Geometry check sheet. Reference: the model listing, model coordinates, mm. Face numbers are marked on the shaded views. A direction names the side the tool comes from. Round coordinates to 2 decimals unless told otherwise and drop trailing zeros. Order: outer loops, then holes, each group sorted by start corner. A loop starts at its lowest first (then second) coordinate and runs counter-clockwise, first axis right, second up. Notation, with made-up numbers: (-23, -9) - (-8, -9) arc R11 cw to (-8, -4) - close; hole circle Ø9 at (17, -17.5). An arc over 180 degrees is marked (long way). Use a Markdown table: item, result. Add a question column.
(1) Section check B-B on z = -10.5. Record the boundary of the cut face in (x, y), then the cut area to 3 significant figures.
(2) Section check C-C on x = -9.5. Record the boundary of the cut face in (y, z), then the cut area to 3 significant figures.
(3) Section check A-A on y = -8.75. Record the boundary of the cut face in (x, z).
(4) Section check D-D on z = -2. Record the boundary of the cut face in (x, y), then the cut area to 3 significant figures.
(5) Access from +Z, -Z, +X, -X, +Y, -Y to the whole of each face (thin tool, end or side, straight path). Record for the marked faces 1, 2, 3, 4 and 5.
(6) Mould release check, pull along X, two halves, no side actions. Record for the marked faces 6, 7 and 8: released by +X, released by -X, zero draft, split by the parting line, or undercut.
(7) Gauge pin test, flat ends, axial feed: P1, Ø11.5, axis at x = 5.5, z = 1, coming from the -Y side; P2, Ø6, axis at x = -13.5, y = -11, coming from the +Z side; P3, Ø5, axis at x = 8, y = -9, coming from the -Z side; P4, Ø5.5, axis at y = -9, z = 10.5, coming from the -X side. Record the tip position at first contact, or that the pin passes through.
(8) Thickness scan on line 1 along X through (y, z) = (-7.5, 11); line 2 along X through (y, z) = (-4, 2). Record the ranges inside material, lowest first. Write a range as [from, to].
```python
from build123d import *

# Parameters (mm, degrees)
F1_DEPTH     = 2.032
F2_DEPTH     = 12.7
F3_T1_DEPTH  = 21.463
F3_T3_DEPTH  = 21.463
F3_T5_DEPTH  = 20.574
F3_T7_DEPTH  = 21.463
F3_T9_DEPTH  = 20.574
F3_T11_DEPTH = 21.463
F3_T17_DEPTH = 27.813
F3_T21_DEPTH = 27.813
F3_T28_DEPTH = 27.813
F3_T32_DEPTH = 27.813
F3_T39_DEPTH = 27.813
F3_T43_DEPTH = 27.813
F3_T50_DEPTH = 27.813
F3_T54_DEPTH = 27.813


# Not quite as in the source:
# - a fillet or chamfer that OpenCascade refuses, or shapes differently, is made with other operations: its cross-section is extruded or revolved along the edge and cut away or added


with BuildPart() as f1:
    # F0 (on Front) → F1 (new body)
    with BuildSketch(Plane.XZ):
        Polygon((1.397, 19.05), (-1.397, 19.05), (-1.397, 1.397), (-19.05, 1.397), (-19.05, -1.397), (-1.397, -1.397), (-1.397, -19.05), (1.397, -19.05), (1.397, -1.397), (19.05, -1.397), (19.05, 1.397), (1.397, 1.397), align=None)
    extrude(amount=F1_DEPTH)

    # F0 (on Front) → F2 (join)
    with BuildSketch(Plane.XZ):
        Polygon((-1.397, 19.05), (-3.937, 19.05), (-3.937, 3.937), (-19.05, 3.937), (-19.05, 1.397), (-1.397, 1.397), align=None)
        Polygon((3.937, 19.05), (1.397, 19.05), (1.397, 1.397), (19.05, 1.397), (19.05, 3.937), (3.937, 3.937), align=None)
        Polygon((-1.397, -1.397), (-19.05, -1.397), (-19.05, -3.937), (-3.937, -3.937), (-3.937, -19.05), (-1.397, -19.05), align=None)
        Polygon((19.05, -3.937), (19.05, -1.397), (1.397, -1.397), (1.397, -19.05), (3.937, -19.05), (3.937, -3.937), align=None)
    extrude(amount=F2_DEPTH)

    # F3: fillet of radius 2.54 on 12 edges, made by hand

    # F3_s2 → F3_t1 (cut)
    with BuildSketch(Plane.XY.offset(3.937)):
        with BuildLine():
            ThreePointArc((-3.937, -2.54), (-3.1930512242, -0.7439487758), (-1.397, 0))
            Line((-1.397, 0), (-3.937, 0))
            Line((-3.937, 0), (-3.937, -2.54))
        make_face()
        with BuildLine():
            ThreePointArc((3.937, -2.54), (3.1930512242, -0.7439487758), (1.397, 0))
            Line((1.397, 0), (3.937, 0))
            Line((3.937, 0), (3.937, -2.54))
        make_face()
    extrude(amount=F3_T1_DEPTH, mode=Mode.SUBTRACT)

    # F3_s4 → F3_t3 (cut)
    with BuildSketch(Plane.YZ.offset(-25.4)):
        with BuildLine():
            ThreePointArc((-2.54, 3.937), (-0.7439487758, 3.1930512242), (0, 1.397))
            Line((0, 1.397), (0, 3.937))
            Line((0, 3.937), (-2.54, 3.937))
        make_face()
        with BuildLine():
            ThreePointArc((-2.54, -3.937), (-0.7439487758, -3.1930512242), (0, -1.397))
            Line((0, -1.397), (0, -3.937))
            Line((0, -3.937), (-2.54, -3.937))
        make_face()
    extrude(amount=F3_T3_DEPTH, mode=Mode.SUBTRACT)

    # F3_s6 → F3_t5 (cut)
    with BuildSketch(Plane.XY.offset(-10.287)):
        with BuildLine():
            ThreePointArc((-19.05, -2.54), (-18.3060512242, -0.7439487758), (-16.51, 0))
            Line((-16.51, 0), (-19.05, 0))
            Line((-19.05, 0), (-19.05, -2.54))
        make_face()
        with BuildLine():
            ThreePointArc((19.05, -2.54), (18.3060512242, -0.7439487758), (16.51, 0))
            Line((16.51, 0), (19.05, 0))
            Line((19.05, 0), (19.05, -2.54))
        make_face()
    extrude(amount=F3_T5_DEPTH, mode=Mode.SUBTRACT)

    # F3_s8 → F3_t7 (cut)
    with BuildSketch(Plane.XY.offset(-25.4)):
        with BuildLine():
            ThreePointArc((-3.937, -2.54), (-3.1930512242, -0.7439487758), (-1.397, 0))
            Line((-1.397, 0), (-3.937, 0))
            Line((-3.937, 0), (-3.937, -2.54))
        make_face()
        with BuildLine():
            ThreePointArc((3.937, -2.54), (3.1930512242, -0.7439487758), (1.397, 0))
            Line((1.397, 0), (3.937, 0))
            Line((3.937, 0), (3.937, -2.54))
        make_face()
    extrude(amount=F3_T7_DEPTH, mode=Mode.SUBTRACT)

    # F3_s10 → F3_t9 (cut)
    with BuildSketch(Plane.YZ.offset(-10.287)):
        with BuildLine():
            ThreePointArc((-2.54, -19.05), (-0.7439487758, -18.3060512242), (0, -16.51))
            Line((0, -16.51), (0, -19.05))
            Line((0, -19.05), (-2.54, -19.05))
        make_face()
        with BuildLine():
            ThreePointArc((-2.54, 19.05), (-0.7439487758, 18.3060512242), (0, 16.51))
            Line((0, 16.51), (0, 19.05))
            Line((0, 19.05), (-2.54, 19.05))
        make_face()
    extrude(amount=F3_T9_DEPTH, mode=Mode.SUBTRACT)

    # F3_s12 → F3_t11 (cut)
    with BuildSketch(Plane.YZ.offset(3.937)):
        with BuildLine():
            ThreePointArc((-2.54, -3.937), (-0.7439487758, -3.1930512242), (0, -1.397))
            Line((0, -1.397), (0, -3.937))
            Line((0, -3.937), (-2.54, -3.937))
        make_face()
        with BuildLine():
            ThreePointArc((-2.54, 3.937), (-0.7439487758, 3.1930512242), (0, 1.397))
            Line((0, 1.397), (0, 3.937))
            Line((0, 3.937), (-2.54, 3.937))
        make_face()
    extrude(amount=F3_T11_DEPTH, mode=Mode.SUBTRACT)


with BuildPart() as f3_tool15:
    # F3_s16 → F3_t17 (new body)
    with BuildSketch(Plane.XY.offset(25.4)):
        with BuildLine():
            ThreePointArc((-3.937, -2.54), (-3.1930512242, -0.7439487758), (-1.397, 0))
            Line((-1.397, 0), (-3.937, 0))
            Line((-3.937, 0), (-3.937, -2.54))
        make_face()
    extrude(amount=-F3_T17_DEPTH)

    split(bisect_by=Plane.XY.offset(3.937), keep=Keep.BOTTOM)


with BuildPart() as f3_tool19:
    # F3_s20 → F3_t21 (new body)
    with BuildSketch(Plane.YZ.offset(2.413)):
        with BuildLine():
            ThreePointArc((-2.54, 3.937), (-0.7439487758, 3.1930512242), (0, 1.397))
            Line((0, 1.397), (0, 3.937))
            Line((0, 3.937), (-2.54, 3.937))
        make_face()
    extrude(amount=-F3_T21_DEPTH)

    split(bisect_by=Plane.YZ.offset(-3.937), keep=Keep.TOP)


with BuildPart() as f3_tool15_1:
    add(f3_tool15.part)

    # F3_t23: intersect F3_tool19
    add(f3_tool19.part, mode=Mode.INTERSECT)


with BuildPart() as f1_1:
    add(f1.part)

    # F3_t13: cut F3_tool15
    add(f3_tool15_1.part, mode=Mode.SUBTRACT)


with BuildPart() as f3_tool26:
    # F3_s27 → F3_t28 (new body)
    with BuildSketch(Plane.YZ.offset(-25.4)):
        with BuildLine():
            ThreePointArc((-2.54, -3.937), (-0.7439487758, -3.1930512242), (0, -1.397))
            Line((0, -1.397), (0, -3.937))
            Line((0, -3.937), (-2.54, -3.937))
        make_face()
    extrude(amount=F3_T28_DEPTH)

    split(bisect_by=Plane.YZ.offset(-3.937), keep=Keep.TOP)


with BuildPart() as f3_tool30:
    # F3_s31 → F3_t32 (new body)
    with BuildSketch(Plane.XY.offset(2.413)):
        with BuildLine():
            ThreePointArc((-3.937, -2.54), (-3.1930512242, -0.7439487758), (-1.397, 0))
            Line((-1.397, 0), (-3.937, 0))
            Line((-3.937, 0), (-3.937, -2.54))
        make_face()
    extrude(amount=-F3_T32_DEPTH)

    split(bisect_by=Plane.XY.offset(-3.937), keep=Keep.TOP)


with BuildPart() as f3_tool26_1:
    add(f3_tool26.part)

    # F3_t34: intersect F3_tool30
    add(f3_tool30.part, mode=Mode.INTERSECT)


with BuildPart() as f1_2:
    add(f1_1.part)

    # F3_t24: cut F3_tool26
    add(f3_tool26_1.part, mode=Mode.SUBTRACT)


with BuildPart() as f3_tool37:
    # F3_s38 → F3_t39 (new body)
    with BuildSketch(Plane.XY.offset(-25.4)):
        with BuildLine():
            ThreePointArc((3.937, -2.54), (3.1930512242, -0.7439487758), (1.397, 0))
            Line((1.397, 0), (3.937, 0))
            Line((3.937, 0), (3.937, -2.54))
        make_face()
    extrude(amount=F3_T39_DEPTH)

    split(bisect_by=Plane.XY.offset(-3.937), keep=Keep.TOP)


with BuildPart() as f3_tool41:
    # F3_s42 → F3_t43 (new body)
    with BuildSketch(Plane.YZ.offset(-2.413)):
        with BuildLine():
            ThreePointArc((-2.54, -3.937), (-0.7439487758, -3.1930512242), (0, -1.397))
            Line((0, -1.397), (0, -3.937))
            Line((0, -3.937), (-2.54, -3.937))
        make_face()
    extrude(amount=F3_T43_DEPTH)

    split(bisect_by=Plane.YZ.offset(3.937), keep=Keep.BOTTOM)


with BuildPart() as f3_tool37_1:
    add(f3_tool37.part)

    # F3_t45: intersect F3_tool41
    add(f3_tool41.part, mode=Mode.INTERSECT)


with BuildPart() as f1_3:
    add(f1_2.part)

    # F3_t35: cut F3_tool37
    add(f3_tool37_1.part, mode=Mode.SUBTRACT)


with BuildPart() as f3_tool48:
    # F3_s49 → F3_t50 (new body)
    with BuildSketch(Plane.YZ.offset(25.4)):
        with BuildLine():
            ThreePointArc((-2.54, 3.937), (-0.7439487758, 3.1930512242), (0, 1.397))
            Line((0, 1.397), (0, 3.937))
            Line((0, 3.937), (-2.54, 3.937))
        make_face()
    extrude(amount=-F3_T50_DEPTH)

    split(bisect_by=Plane.YZ.offset(3.937), keep=Keep.BOTTOM)


with BuildPart() as f3_tool52:
    # F3_s53 → F3_t54 (new body)
    with BuildSketch(Plane.XY.offset(-2.413)):
        with BuildLine():
            ThreePointArc((3.937, -2.54), (3.1930512242, -0.7439487758), (1.397, 0))
            Line((1.397, 0), (3.937, 0))
            Line((3.937, 0), (3.937, -2.54))
        make_face()
    extrude(amount=F3_T54_DEPTH)

    split(bisect_by=Plane.XY.offset(3.937), keep=Keep.BOTTOM)


with BuildPart() as f3_tool48_1:
    add(f3_tool48.part)

    # F3_t56: intersect F3_tool52
    add(f3_tool52.part, mode=Mode.INTERSECT)


with BuildPart() as f1_4:
    add(f1_3.part)

    # F3_t46: cut F3_tool48
    add(f3_tool48_1.part, mode=Mode.SUBTRACT)


solid = f1_4.part
```
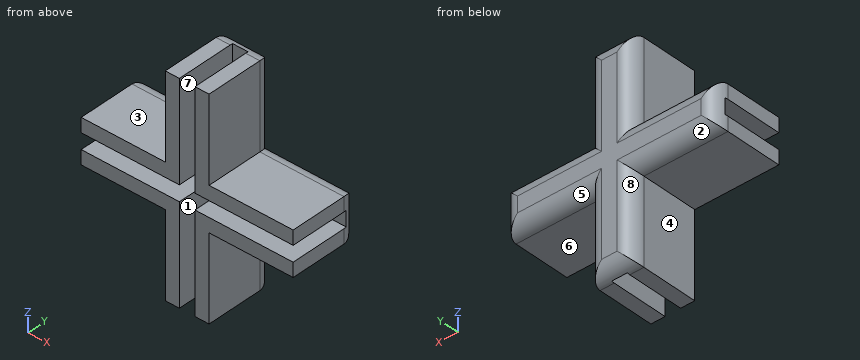
Check sheet entries:
| question | item | result |
|---|---|---|
| 1 | outline | (-3.94, -12.7) - (-1.4, -12.7) - (-1.4, -2.03) - (1.4, -2.03) - (1.4, -12.7) - (3.94, -12.7) - (3.94, -2.54) arc R2.54 ccw to (1.4, 0) - (-1.4, 0) arc R2.54 ccw to (-3.94, -2.54) - close |
| 1 | area | 67.4 mm2 |
| 2 | outline | (-12.7, -3.94) - (-2.54, -3.94) arc R2.54 ccw to (0, -1.4) - (0, 1.4) arc R2.54 ccw to (-2.54, 3.94) - (-12.7, 3.94) - (-12.7, 1.4) - (-2.03, 1.4) - (-2.03, -1.4) - (-12.7, -1.4) - close |
| 2 | area | 67.4 mm2 |
| 3 | outline | (-19.05, -3.94) - (-3.94, -3.94) - (-3.94, -19.05) - (-1.4, -19.05) - (-1.4, -1.4) - (-19.05, -1.4) - close; (-19.05, 1.4) - (-1.4, 1.4) - (-1.4, 19.05) - (-3.94, 19.05) - (-3.94, 3.94) - (-19.05, 3.94) - close; (1.4, -19.05) - (3.94, -19.05) - (3.94, -3.94) - (19.05, -3.94) - (19.05, -1.4) - (1.4, -1.4) - close; (1.4, 1.4) - (19.05, 1.4) - (19.05, 3.94) - (3.94, 3.94) - (3.94, 19.05) - (1.4, 19.05) - close |
| 4 | outline | (-19.05, -12.7) - (-1.4, -12.7) - (-1.4, -2.03) - (1.4, -2.03) - (1.4, -12.7) - (19.05, -12.7) - (19.05, -2.54) arc R2.54 ccw to (17.11, -0.07) - (2, -0.07) arc R2.54 ccw to (1.4, 0) - (-1.4, 0) arc R2.54 ccw to (-2, -0.07) - (-17.11, -0.07) arc R2.54 ccw to (-19.05, -2.54) - close |
| 4 | area | 449 mm2 |
| 5 | face 1 | +Z, -Z, -Y |
| 5 | face 2 | -Z, -X, +Y |
| 5 | face 3 | +Z, -X, +Y, -Y |
| 5 | face 4 | -Z, -X, +Y, -Y |
| 5 | face 5 | -Z, +X, +Y |
| 6 | face 6 | zero draft |
| 6 | face 7 | undercut |
| 6 | face 8 | released by -X |
| 7 | P1 | stops at y = -12.7 |
| 7 | P2 | stops at z = 3.94 |
| 7 | P3 | stops at z = -3.94 |
| 7 | P4 | stops at x = -3.94 |
| 8 | line 1 | x = [-3.94, -1.4], [1.4, 3.94] |
| 8 | line 2 | x = [-19.05, -1.4], [1.4, 19.05] |
